from build123d import *

# Parameters (mm, degrees)
F0_R         = 7.62
F1_DEPTH     = 19.05
F3_DEPTH     = 12.7
F4_SIZE      = 1.27
F5_T1_DEPTH  = 8.5497045256
F5_T3_DEPTH  = 8.5497045256
F5_T5_DEPTH  = 8.5497045256
F5_T7_DEPTH  = 8.5497045256
F5_T12_DEPTH = 8.5497045256
F5_S13_R     = 7.62
F5_T14_DEPTH = 6
F5_T18_DEPTH = 8.5497045256
F5_S19_R     = 7.62
F5_T20_DEPTH = 6
F5_T24_DEPTH = 8.5497045256
F5_S25_R     = 7.62
F5_T26_DEPTH = 6
F5_T30_DEPTH = 8.5497045256
F5_S31_R     = 7.62
F5_T32_DEPTH = 6
F5_T36_DEPTH = 8.5497045256
F5_S37_R     = 7.62
F5_T38_DEPTH = 6
F5_T42_DEPTH = 8.5497045256
F5_S43_R     = 7.62
F5_T44_DEPTH = 6
F6_R         = 7.14375
F7_DEPTH     = 12.7
F8_R         = 6.35
F9_DEPTH     = 44.4510001


# Not quite as in the source:
# - a fillet or chamfer that OpenCascade refuses, or shapes differently, is made with other operations: its cross-section is extruded or revolved along the edge and cut away or added


with BuildPart() as f1:
    # F0 (on Front) → F1 (new body)
    with BuildSketch(Plane.XZ):
        Circle(F0_R)
    extrude(amount=F1_DEPTH)

    # F2 (on face) → F3 (join)
    with BuildSketch(Plane.XZ.offset(19.05)):
        with BuildLine():
            Line((7.8629215405, 3.9488814679), (4.1872753391, 6.3664059904))
            ThreePointArc((4.1872753391, 6.3664059904), (6.7071394083, 3.6164459015), (7.62, 0))
            ThreePointArc((7.62, 0), (7.616776064, -0.2216357159), (7.6071069841, -0.4430838887))
            Line((7.6071069841, -0.4430838887), (7.8629215405, 3.9488814679))
        make_face()
        with BuildLine():
            ThreePointArc((4.1872753391, 6.3664059904), (0.4430838236, 7.6071069879), (-3.4198316443, 6.8094898138))
            ThreePointArc((-3.4198316443, 6.8094898138), (-6.3664059346, 4.187275424), (-7.6071069765, 0.4430840189))
            ThreePointArc((-7.6071069765, 0.4430840189), (-6.8094898664, -3.4198315396), (-4.187275378, -6.3664059648))
            ThreePointArc((-4.187275378, -6.3664059648), (-0.4430838337, -7.6071069873), (3.419831668, -6.8094898019))
            ThreePointArc((3.419831668, -6.8094898019), (6.3664059777, -4.1872753585), (7.6071069841, -0.4430838887))
            ThreePointArc((7.6071069841, -0.4430838887), (7.616776064, -0.2216357159), (7.62, 0))
            ThreePointArc((7.62, 0), (6.7071394083, 3.6164459015), (4.1872753391, 6.3664059904))
        make_face()
        with BuildLine():
            ThreePointArc((7.6071069841, -0.4430838887), (6.3664059777, -4.1872753585), (3.419831668, -6.8094898019))
            Line((3.419831668, -6.8094898019), (7.351292438, -4.8350490681))
            Line((7.351292438, -4.8350490681), (7.6071069841, -0.4430838887))
        make_face()
        with BuildLine():
            ThreePointArc((3.419831668, -6.8094898019), (-0.4430838337, -7.6071069873), (-4.187275378, -6.3664059648))
            Line((-4.187275378, -6.3664059648), (-0.5116291025, -8.783930536))
            Line((-0.5116291025, -8.783930536), (3.419831668, -6.8094898019))
        make_face()
        with BuildLine():
            ThreePointArc((-4.187275378, -6.3664059648), (-6.8094898664, -3.4198315396), (-7.6071069765, 0.4430840189))
            Line((-7.6071069765, 0.4430840189), (-7.8629215405, -3.9488814679))
            Line((-7.8629215405, -3.9488814679), (-4.187275378, -6.3664059648))
        make_face()
        with BuildLine():
            Line((-3.4198316443, 6.8094898138), (-7.351292438, 4.8350490681))
            Line((-7.351292438, 4.8350490681), (-7.6071069765, 0.4430840189))
            ThreePointArc((-7.6071069765, 0.4430840189), (-6.3664059346, 4.187275424), (-3.4198316443, 6.8094898138))
        make_face()
        with BuildLine():
            Line((0.5116291025, 8.783930536), (-3.4198316443, 6.8094898138))
            ThreePointArc((-3.4198316443, 6.8094898138), (0.4430838236, 7.6071069879), (4.1872753391, 6.3664059904))
            Line((4.1872753391, 6.3664059904), (0.5116291025, 8.783930536))
        make_face()
    extrude(amount=F3_DEPTH)

    # F4
    f4_edges = [f1.edges().sort_by_distance(p)[0] for p in [
        (7.862922, -25.4, 3.948881),
        (7.351292, -25.4, -4.835049),
        (-0.511629, -25.4, -8.783931),
        (-7.862922, -25.4, -3.948881),
        (-7.351292, -25.4, 4.835049),
        (0.511629, -25.4, 8.783931),
    ]]
    chamfer(f4_edges, length=F4_SIZE)

    # F5: fillet of radius 1.27 on 12 edges, made by hand

    # F5_s2 → F5_t1 (cut)
    with BuildSketch(Plane(origin=(1.918540045, 0, -3.8201526101), x_dir=(0, 1, 0), z_dir=(-0.4487968068, 0, 0.8936338323))):
        with BuildLine():
            ThreePointArc((-30.48, -8.1638181024), (-31.3780256121, -7.7918437146), (-31.75, -6.8938181024))
            Line((-31.75, -6.8938181024), (-31.75, -8.1638181024))
            Line((-31.75, -8.1638181024), (-30.48, -8.1638181024))
        make_face()
        with BuildLine():
            ThreePointArc((-31.75, 6.8938181024), (-31.3780256121, 7.7918437146), (-30.48, 8.1638181024))
            Line((-30.48, 8.1638181024), (-31.75, 8.1638181024))
            Line((-31.75, 8.1638181024), (-31.75, 6.8938181024))
        make_face()
    extrude(amount=F5_T1_DEPTH, mode=Mode.SUBTRACT)

    # F5_s4 → F5_t3 (cut)
    with BuildSketch(Plane(origin=(4.2676192292, 0, -0.2485718879), x_dir=(0, 1, 0), z_dir=(-0.9983080038, 0, 0.0581474803))):
        with BuildLine():
            ThreePointArc((-31.75, -6.8938181024), (-31.3780256121, -7.7918437146), (-30.48, -8.1638181024))
            Line((-30.48, -8.1638181024), (-31.75, -8.1638181024))
            Line((-31.75, -8.1638181024), (-31.75, -6.8938181024))
        make_face()
        with BuildLine():
            ThreePointArc((-31.75, 6.8938181024), (-31.3780256121, 7.7918437146), (-30.48, 8.1638181024))
            Line((-30.48, 8.1638181024), (-31.75, 8.1638181024))
            Line((-31.75, 8.1638181024), (-31.75, 6.8938181024))
        make_face()
    extrude(amount=F5_T3_DEPTH, mode=Mode.SUBTRACT)

    # F5_s6 → F5_t5 (cut)
    with BuildSketch(Plane(origin=(-2.3490791841, 0, -3.5715807222), x_dir=(0, 1, 0), z_dir=(0.5495111971, 0, 0.835486352))):
        with BuildLine():
            ThreePointArc((-31.75, 6.8938181024), (-31.3780256121, 7.7918437146), (-30.48, 8.1638181024))
            Line((-30.48, 8.1638181024), (-31.75, 8.1638181024))
            Line((-31.75, 8.1638181024), (-31.75, 6.8938181024))
        make_face()
    extrude(amount=F5_T5_DEPTH, mode=Mode.SUBTRACT)

    # F5_s8 → F5_t7 (cut)
    with BuildSketch(Plane(origin=(2.3490791841, 0, 3.5715807222), x_dir=(0, 1, 0), z_dir=(-0.5495111971, 0, -0.835486352))):
        with BuildLine():
            ThreePointArc((-30.48, 8.1638181024), (-31.3780256121, 7.7918437146), (-31.75, 6.8938181024))
            Line((-31.75, 6.8938181024), (-31.75, 8.1638181024))
            Line((-31.75, 8.1638181024), (-30.48, 8.1638181024))
        make_face()
    extrude(amount=F5_T7_DEPTH, mode=Mode.SUBTRACT)


with BuildPart() as f5_tool10:
    # F5_s11 → F5_t12 (new body)
    with BuildSketch(Plane(origin=(4.2676192292, 0, -0.2485718879), x_dir=(0, 1, 0), z_dir=(-0.9983080038, 0, 0.0581474803))):
        with BuildLine():
            ThreePointArc((-19.05, -6.8938181024), (-19.4219743879, -7.7918437146), (-20.32, -8.1638181024))
            Line((-20.32, -8.1638181024), (-19.05, -8.1638181024))
            Line((-19.05, -8.1638181024), (-19.05, -6.8938181024))
        make_face()
    extrude(amount=F5_T12_DEPTH)

    # F5_s13 → F5_t14 (cut, symmetric)
    with BuildSketch(Plane.XZ.offset(19.7)):
        Circle(F5_S13_R)
    extrude(amount=F5_T14_DEPTH, both=True, mode=Mode.SUBTRACT)


with BuildPart() as f1_1:
    add(f1.part)

    # F5_t9: cut F5_tool10
    add(f5_tool10.part, mode=Mode.SUBTRACT)


with BuildPart() as f5_tool16:
    # F5_s17 → F5_t18 (new body)
    with BuildSketch(Plane(origin=(-2.3490791841, 0, -3.5715807222), x_dir=(0, 1, 0), z_dir=(0.5495111971, 0, 0.835486352))):
        with BuildLine():
            ThreePointArc((-19.05, 6.8938181024), (-19.4219743879, 7.7918437146), (-20.32, 8.1638181024))
            Line((-20.32, 8.1638181024), (-19.05, 8.1638181024))
            Line((-19.05, 8.1638181024), (-19.05, 6.8938181024))
        make_face()
    extrude(amount=F5_T18_DEPTH)

    # F5_s19 → F5_t20 (cut, symmetric)
    with BuildSketch(Plane.XZ.offset(19.7)):
        Circle(F5_S19_R)
    extrude(amount=F5_T20_DEPTH, both=True, mode=Mode.SUBTRACT)


with BuildPart() as f1_2:
    add(f1_1.part)

    # F5_t15: cut F5_tool16
    add(f5_tool16.part, mode=Mode.SUBTRACT)


with BuildPart() as f5_tool22:
    # F5_s23 → F5_t24 (new body)
    with BuildSketch(Plane(origin=(1.918540045, 0, -3.8201526101), x_dir=(0, 1, 0), z_dir=(-0.4487968068, 0, 0.8936338323))):
        with BuildLine():
            ThreePointArc((-19.05, 6.8938181024), (-19.4219743879, 7.7918437146), (-20.32, 8.1638181024))
            Line((-20.32, 8.1638181024), (-19.05, 8.1638181024))
            Line((-19.05, 8.1638181024), (-19.05, 6.8938181024))
        make_face()
    extrude(amount=F5_T24_DEPTH)

    # F5_s25 → F5_t26 (cut, symmetric)
    with BuildSketch(Plane.XZ.offset(19.7)):
        Circle(F5_S25_R)
    extrude(amount=F5_T26_DEPTH, both=True, mode=Mode.SUBTRACT)


with BuildPart() as f1_3:
    add(f1_2.part)

    # F5_t21: cut F5_tool22
    add(f5_tool22.part, mode=Mode.SUBTRACT)


with BuildPart() as f5_tool28:
    # F5_s29 → F5_t30 (new body)
    with BuildSketch(Plane(origin=(4.2676192292, 0, -0.2485718879), x_dir=(0, 1, 0), z_dir=(-0.9983080038, 0, 0.0581474803))):
        with BuildLine():
            ThreePointArc((-19.05, 6.8938181024), (-19.4219743879, 7.7918437146), (-20.32, 8.1638181024))
            Line((-20.32, 8.1638181024), (-19.05, 8.1638181024))
            Line((-19.05, 8.1638181024), (-19.05, 6.8938181024))
        make_face()
    extrude(amount=F5_T30_DEPTH)

    # F5_s31 → F5_t32 (cut, symmetric)
    with BuildSketch(Plane.XZ.offset(19.7)):
        Circle(F5_S31_R)
    extrude(amount=F5_T32_DEPTH, both=True, mode=Mode.SUBTRACT)


with BuildPart() as f1_4:
    add(f1_3.part)

    # F5_t27: cut F5_tool28
    add(f5_tool28.part, mode=Mode.SUBTRACT)


with BuildPart() as f5_tool34:
    # F5_s35 → F5_t36 (new body)
    with BuildSketch(Plane(origin=(2.3490791841, 0, 3.5715807222), x_dir=(0, 1, 0), z_dir=(-0.5495111971, 0, -0.835486352))):
        with BuildLine():
            ThreePointArc((-19.05, 6.8938181024), (-19.4219743879, 7.7918437146), (-20.32, 8.1638181024))
            Line((-20.32, 8.1638181024), (-19.05, 8.1638181024))
            Line((-19.05, 8.1638181024), (-19.05, 6.8938181024))
        make_face()
    extrude(amount=F5_T36_DEPTH)

    # F5_s37 → F5_t38 (cut, symmetric)
    with BuildSketch(Plane.XZ.offset(19.7)):
        Circle(F5_S37_R)
    extrude(amount=F5_T38_DEPTH, both=True, mode=Mode.SUBTRACT)


with BuildPart() as f1_5:
    add(f1_4.part)

    # F5_t33: cut F5_tool34
    add(f5_tool34.part, mode=Mode.SUBTRACT)


with BuildPart() as f5_tool40:
    # F5_s41 → F5_t42 (new body)
    with BuildSketch(Plane(origin=(1.918540045, 0, -3.8201526101), x_dir=(0, 1, 0), z_dir=(-0.4487968068, 0, 0.8936338323))):
        with BuildLine():
            ThreePointArc((-19.05, -6.8938181024), (-19.4219743879, -7.7918437146), (-20.32, -8.1638181024))
            Line((-20.32, -8.1638181024), (-19.05, -8.1638181024))
            Line((-19.05, -8.1638181024), (-19.05, -6.8938181024))
        make_face()
    extrude(amount=F5_T42_DEPTH)

    # F5_s43 → F5_t44 (cut, symmetric)
    with BuildSketch(Plane.XZ.offset(19.7)):
        Circle(F5_S43_R)
    extrude(amount=F5_T44_DEPTH, both=True, mode=Mode.SUBTRACT)


with BuildPart() as f1_6:
    add(f1_5.part)

    # F5_t39: cut F5_tool40
    add(f5_tool40.part, mode=Mode.SUBTRACT)

    # F6 (on face) → F7 (join)
    with BuildSketch(Plane.XZ.offset(31.75)):
        Circle(F6_R)
    extrude(amount=F7_DEPTH)

    # F8 (on face) → F9 (cut, through all)
    with BuildSketch(Plane.XZ.offset(44.45)):
        Circle(F8_R)
    extrude(amount=-F9_DEPTH, mode=Mode.SUBTRACT)


solid = f1_6.part
Verification items for the finished model (mm, model axes). A direction names the side the tool comes from. Round coordinates to 2 decimals unless told otherwise and drop trailing zeros. Loops run counter-clockwise (first coordinate to the right, second up) from the corner with the lowest first, then second, coordinate; pieces in that order, holes last. Notation, with made-up numbers: (4.5, 86.25) - (41.5, 86.25) arc R16 cw to (41.5, 104.25) - close; hole circle Ø3 at (-30, 23). An arc over 180 degrees is marked (long way). Write item = value, one per line.
Q1. Tool access check on faces 1 (the flat face through (3.33, -31.75, -6.53)), 2 (the cylindrical face through (-7.137, -38.011, 0.314)), 3 (the flat face through (-4, -31.75, -6.1)). Record the directions out of +Z, -Z, +X, -X, +Y, -Y that give a thin tool (end or side, any length) a straight path to the whole face; none if there is none.
Here are the results:
face_1 = -Z, +X, -Y
face_2 = -Y
face_3 = -Z, -X, -Y
Q2. Depth check by flat-ended pin: pin 1 (1.5 mm diameter, centred on y = -31.5, z = 0.5, fed in from +X); pin 2 (4 mm diameter, centred on y = -33.5, z = -2.5, fed in from -X); pin 3 (8 mm diameter, centred on x = 2, z = -5, fed in from +Y); pin 4 (1.5 mm diameter, centred on y = -13, z = -1.5, fed in from +X). Enter the tip coordinate at first touch or a pass-through.
Here are the results:
pin_1 = 7.71
pin_2 = -7.45
pin_3 = 0
pin_4 = 7.58
Q3. Sectioned sample at A-A on y = -23.5. Record the boundary of the cut face in (x, z), plus the area to 3 significant figures.
Here are the results:
outline = (-7.79, -2.68) - (-6.8, -4.65) - (-1.57, -8.09) - (0.62, -8.21) - (6.22, -5.41) - (7.43, -3.57) - (7.79, 2.68) - (6.8, 4.65) - (1.57, 8.09) - (-0.62, 8.21) - (-6.22, 5.41) - (-7.43, 3.57) - close; hole circle Ø12.7 at (0, 0)
area = 70.3 mm^2
Q4. Material ranges on L1, parallel to Z at x = 0, y = -17.5; L2, parallel to Z at x = 0, y = -32; L3, parallel to X at y = -35, z = -5.25, recorded low to high.
Here are the results:
L1 = -7.62 to -6.35, 6.35 to 7.62
L2 = -7.14 to -6.35, 6.35 to 7.14
L3 = -4.84 to -3.57, 3.57 to 4.84
Q5. Sectioned sample at B-B on y = -13. Record the boundary of the cut face in (x, z).
Here are the results:
outline = circle Ø15.24 at (0, 0); hole circle Ø12.7 at (0, 0)
